Autodesk Inventor part; units mm, degrees
ref_plane "YZ Plane" through (0, 0, 0) normal (1, 0, 0) x (0, 1, 0)
ref_plane "XZ Plane" through (0, 0, 0) normal (0, 1, 0) x (-1, 0, 0)
ref_plane "XY Plane" through (0, 0, 0) normal (0, 0, 1) x (1, 0, 0)
sketch "スケッチ1" plane through (0, 0, 0) normal (0, 1, 0) x (-1, 0, 0)
  line L0 (-3, 9) -> (16, 9)
  line L1 (10, -9) -> (-3, -9)
  line L2 (-5, -7) -> (-5, 7)
  line L3 (16, -20) -> (12, -20)
  line L4 (10, -18) -> (10, -9)
  arc A0 (16, -20) -> (18, -18) centre (16, -18) ccw
  arc A1 (10, -18) -> (12, -20) centre (12, -18) ccw
  arc A2 (-5, -7) -> (-3, -9) centre (-3, -7) ccw
  arc A3 (-3, 9) -> (-5, 7) centre (-3, 7) ccw
  line L5 (18, 7) -> (18, -18)
  arc A4 (18, 7) -> (16, 9) centre (16, 7) ccw
  point P0 (0, 0)
  point P1 (-5, 9)
  point P2 (-5, -9)
  point P3 (18, -20)
  point P4 (10, -20)
  point P5 (10, 9)
  point P6 (18, 9)
  dimension "d0" = 5
  dimension "d4" = 18
  dimension "d5" = 9
  dimension "d7" = 20
  dimension "d8" = 10
  dimension "d40" = 2
extrude "プレート1" add sketch "スケッチ1" along normal blind 3
sketch "スケッチ3" plane through (0, 3, 0) normal (0, 1, 0) x (1, 0, 0)
  line L0 (-10, 18) -> (-10, 9)
  line L1 (-16, 20) -> (-12, 20)
  line L2 (-18, -7) -> (-18, 18)
  line L3 (-10, 9) -> (3, 9)
  line L4 (3, -9) -> (-16, -9)
  point P0 (-14, 16)
  point P1 (-14, 0)
  dimension "d42" = 4
  dimension "d43" = 4
  dimension "d44" = 4
  dimension "d45" = 18
  dimension "d46" = 9
hole "穴3" at (1, 3, 0) direction (0, -1, 0) diameter 4.2 end through all
sketch "スケッチ2" plane through (0, 0, 0) normal (0, -1, 0) x (1, 0, 0)
  circle A0 centre (1, 0) radius 2.1
  line L0 (3, 9) -> (-16, 9)
  arc A1 (-18, -18) -> (-16, -20) centre (-16, -18) ccw
  line L1 (-16, -20) -> (-12, -20)
  arc A2 (-12, -20) -> (-10, -18) centre (-12, -18) ccw
  line L2 (-10, -18) -> (-10, -9)
  line L3 (-10, -9) -> (3, -9)
  arc A3 (3, -9) -> (5, -7) centre (3, -7) ccw
  line L4 (5, -7) -> (5, 7)
  arc A4 (5, 7) -> (3, 9) centre (3, 7) ccw
  line L5 (-18, 7) -> (-18, -18)
  arc A5 (-16, 9) -> (-18, 7) centre (-16, 7) ccw
  point P0 (0, 0)
fillet "フィレット1" radius 2.5 1 edges at (-10, 1.5, -9)
hole "穴4" at (-14, 3, -16) at (-14, 3, 0) direction (0, -1, 0) diameter 4.2 end through all
equation "\"d37\" = Thickness"
equation "\"d52\" = Thickness"
equation "\"d9\" = Thickness"
equation "\"BendRadius\" = Thickness"
equation "\"BendReliefWidth\" = Thickness"
equation "\"BendReliefDepth\" = 0.5 * Thickness"
equation "\"CornerReliefSize\" = 4 * Thickness"
equation "\"MinimumRemnant\" = 2 * Thickness"
equation "\"TransitionRadius\" = BendRadius"
equation "\"JacobiRadiusSize\" = BendRadius"
equation "\"GapSize\" = Thickness"
properties part number "L_almite_braket"
Input: part model. Units: mm. Frame: model coordinates. A direction names the side the tool comes from. Give positions to 0.01 mm unless a question says otherwise; leave off trailing zeros. Loops run counter-clockwise (first coordinate to the right, second up) from the corner with the lowest first, then second, coordinate; pieces in that order, holes last. Notation, with made-up numbers: (66, -14) -> (125, -14) arc R25 ccw to (125, 4) -> close; hole circle Ø7 at (22, 82.5). An arc over 180 degrees is marked (long way). Use a Markdown table: item, result.
Q1. Pull-direction query (X, two-part tool) for faces 3 (the flat face through (-6, 1, 9)), 4 (the cylindrical face through (-14.09, 1.48, -2.1)), 5 (the cylindrical face through (-10.6, 1.48, -19.43)), 6 (the cylindrical face through (-14.09, 1.48, -18.1)); classes: pulls with the +X half, pulls with the -X half, needs draft (parallel to the pull), parting line crosses it, or undercut.
Entries:
| item | result |
|---|---|
| face 3 | needs draft |
| face 4 | undercut |
| face 5 | pulls with the +X half |
| face 6 | undercut |
Q2. First-contact query: P1, Ø2.5, axis at x = -14, z = 0, coming from the -Y side; P2, Ø1.5, axis at x = -4.5, y = 2, coming from the -Z side; P3, Ø1.5, axis at y = 1, z = -16, coming from the +X side. Flat tips, straight axial feed; report the tip coordinate or a pass-through.
Entries:
| item | result |
|---|---|
| P1 | passes through |
| P2 | stops at z = -9 |
| P3 | stops at x = -10 |
Q3. Section query D-D, the plane x = 1. Return the cut outline in (y, z).
Entries:
| item | result |
|---|---|
| outline | (0, -9) -> (3, -9) -> (3, -2.1) -> (0, -2.1) -> close; (0, 2.1) -> (3, 2.1) -> (3, 9) -> (0, 9) -> close |
Q4. Section query C-C, the plane y = 2. Return the cut outline in (x, z), plus the area to 3 significant figures.
Entries:
| item | result |
|---|---|
| outline | (-18, -18) arc R2 ccw to (-16, -20) -> (-12, -20) arc R2 ccw to (-10, -18) -> (-10, -11.5) arc R2.5 cw to (-7.5, -9) -> (3, -9) arc R2 ccw to (5, -7) -> (5, 7) arc R2 ccw to (3, 9) -> (-16, 9) arc R2 ccw to (-18, 7) -> close; hole circle Ø4.2 at (-14, -16); hole circle Ø4.2 at (-14, 0); hole circle Ø4.2 at (1, 0) |
| area | 457 mm² |
Q5. Access query for faces 1 (the flat face through (-2, 1, -9)), 2 (the cylindrical face through (-17.43, 1.48, -19.4)). Directions: +Z, -Z, +X, -X, +Y, -Y. A direction counts if a zero-diameter tool reaches every point of the face in a straight line with its end or side. Return the directions, or none.
Entries:
| item | result |
|---|---|
| face 1 | -Z, +X, +Y, -Y |
| face 2 | -Z, -X, +Y, -Y |
Q6. Section query A-A, the plane x = -14. Return the cut outline in (y, z), plus the area to 3 significant figures.
Entries:
| item | result |
|---|---|
| outline | (0, -20) -> (3, -20) -> (3, -18.1) -> (0, -18.1) -> close; (0, -13.9) -> (3, -13.9) -> (3, -2.1) -> (0, -2.1) -> close; (0, 2.1) -> (3, 2.1) -> (3, 9) -> (0, 9) -> close |
| area | 61.8 mm² |
Q7. Section query B-B, the plane z = 0. Return the cut outline in (x, y).
Entries:
| item | result |
|---|---|
| outline | (-18, 0) -> (-16.1, 0) -> (-16.1, 3) -> (-18, 3) -> close; (-11.9, 0) -> (-1.1, 0) -> (-1.1, 3) -> (-11.9, 3) -> close; (3.1, 0) -> (5, 0) -> (5, 3) -> (3.1, 3) -> close |
Q8. Ray query, probe 1 along Z at (x, y) = (-14, 1); probe 2 along X at (y, z) = (0.7, 0); probe 3 along X at (y, z) = (2.05, -16). Return the intervals inside material, ascending. Write a range as from..to.
Entries:
| item | result |
|---|---|
| probe 1 | z = -20..-18.1, -13.9..-2.1, 2.1..9 |
| probe 2 | x = -18..-16.1, -11.9..-1.1, 3.1..5 |
| probe 3 | x = -18..-16.1, -11.9..-10 |
